Part print with two shaded views. Sizes in mm from the minimum x, y, z corner. Give positions to 0.01 mm unless a question says otherwise; leave off trailing zeros. Write each loop counter-clockwise with the first axis right and the second up, starting at its lowest first coordinate (ties: lowest second). Pieces come first, ordered by that corner, then holes. Notation, with made-up numbers: M -28.75,21 L 4.25,21 A25 cw 4.25,34 Z; hole C 75,61.5 d9. An arc over 180 degrees is marked long. Return JSON: item names as keys, results as strings. Group by question number.
Q1. Flat gauge pins, fed straight in: pin 1 Ø5 at (x, z) = (47.5, 64.5) entering from -Y; pin 2 Ø8 at (x, y) = (34, 35) entering from -Z; pin 3 Ø11 at (x, z) = (5, 33) entering from +Y. Where does each tip first touch, or does it go through?
Q2. Band-saw the part on A-A, the plane z = 37. Give the cut face in (x, y).
Q3. Wall check: probe 1 along X at (y, z) = (35, 40.5); probe 2 along Z at (x, y) = (11, 12); probe 3 along Z at (x, y) = (49, 32). Give the ranges that are in metal, low to high.
Q4. Band-saw the part on D-D, the plane x = 35. Give the cut face in (y, z).
Q5. Band-saw the part on B-B, the plane x = 4.5. Give the cut face in (y, z), then the cut area to 3 significant figures.
Q6. Band-saw the part on C-C, the plane y = 24. Give the cut face in (x, z), then the cut area to 3 significant figures.
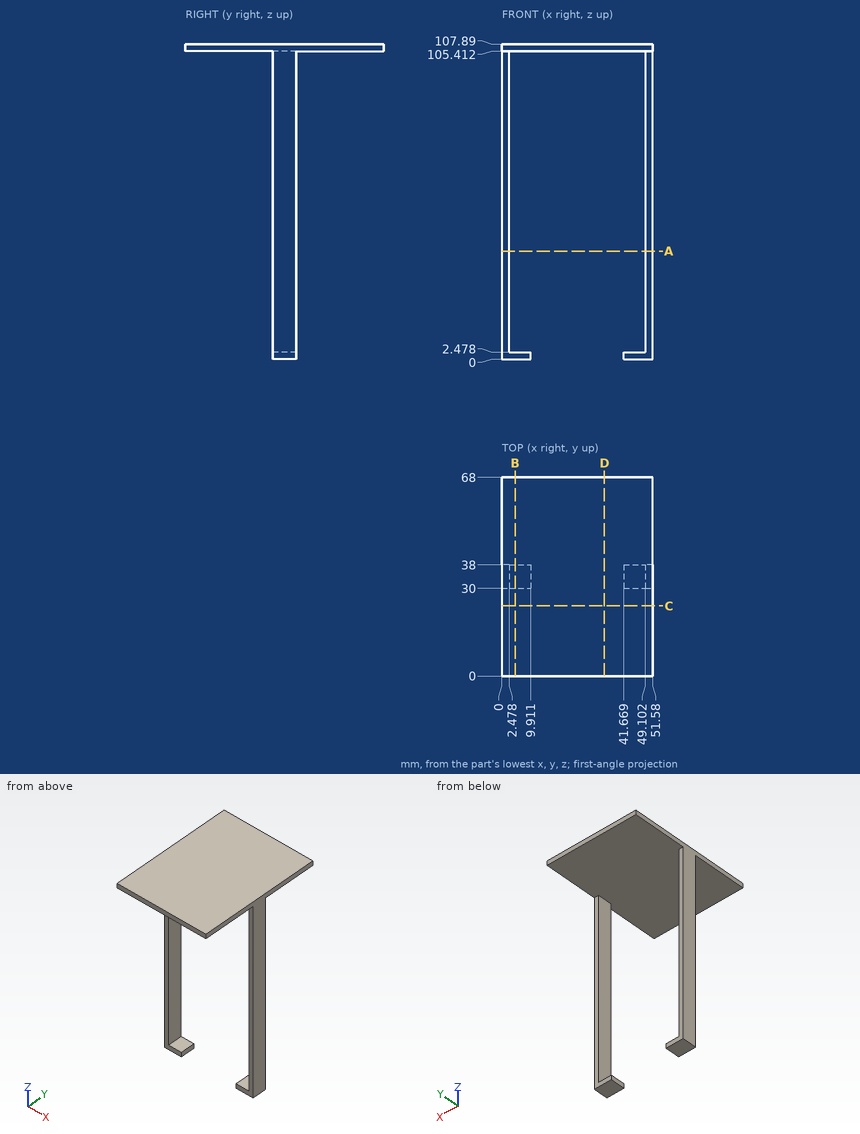
From the geometry:
{
 "1": {"pin 1": "stops at y = 30", "pin 2": "stops at z = 105.41", "pin 3": "stops at y = 38"},
 "2": {"outline": "M 0,30 L 2.48,30 L 2.48,38 L 0,38 Z; M 49.1,30 L 51.58,30 L 51.58,38 L 49.1,38 Z"},
 "3": {"probe 1": "x = 0 to 2.48, 49.1 to 51.58", "probe 2": "z = 105.41 to 107.89", "probe 3": "z = 0 to 2.48, 105.41 to 107.89"},
 "4": {"outline": "M 0,105.41 L 68,105.41 L 68,107.89 L 0,107.89 Z"},
 "5": {"outline": "M 0,105.41 L 68,105.41 L 68,107.89 L 0,107.89 Z; M 30,0 L 38,0 L 38,2.48 L 30,2.48 Z", "area": "188 mm^2"},
 "6": {"outline": "M 0,105.41 L 51.58,105.41 L 51.58,107.89 L 0,107.89 Z", "area": "128 mm^2"}
}
